Check sheet for the modelled part. Datum: model origin and axes. Units: mm. Face numbers are marked on the shaded views. A direction names the side the tool comes from. Round coordinates to 2 decimals unless told otherwise and drop trailing zeros. Write each loop counter-clockwise with the first axis right and the second up, starting at its lowest first coordinate (ties: lowest second). Pieces come first, ordered by that corner, then holes. Notation, with made-up numbers: (-20, -35.5) -> (34, -35.5) arc R19 ccw to (34, -11.5) -> close; hole circle Ø7 at (-21.75, 86). An arc over 180 degrees is marked (long way). One line per item, written item: value.
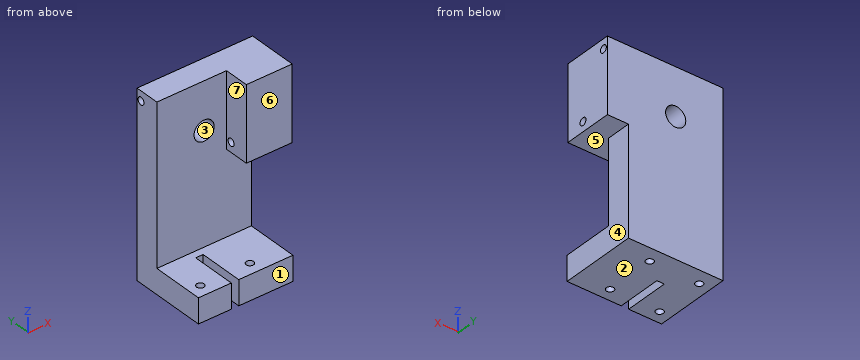
from build123d import *

# Parameters (mm, degrees)
SKETCH1_W                = 38.1
SKETCH1_H                = 63.5
SKETCH1_R                = 4.064
BOSS_EXTRUDE1_DEPTH      = 10
BOSS_EXTRUDE2_DEPTH      = 8.5
BOSS_EXTRUDE2_DEPTH_BACK = 10
BOSS_EXTRUDE2_START      = 38.1
SKETCH2_R                = 1.5
SKETCH3_R                = 1.5
BOSS_EXTRUDE3_DEPTH      = 10
SKETCH2_2_R              = 1.5
CUT_EXTRUDE1_DEPTH       = 10
CUT_EXTRUDE2_START       = 10
SKETCH3_2_R              = 1.5
CUT_EXTRUDE2_DEPTH       = 10


with BuildPart() as part:
    # Sketch1 → Boss-Extrude1 (new body)
    with BuildSketch(Plane(origin=(0, 0, 0), x_dir=(1, 0, 0), z_dir=(0, 1, 0))):
        with Locations((19.05, -31.75)):
            Rectangle(SKETCH1_W, SKETCH1_H)
        with Locations(Location((19.05, -44.45, 0), (0, 0, 270))):
            Circle(SKETCH1_R, mode=Mode.SUBTRACT)
    extrude(amount=BOSS_EXTRUDE1_DEPTH)

    # Sketch2 → Boss-Extrude2 (add, two sides: drawn at the far end of the back side and taken through both)
    with BuildSketch(Plane(origin=(0, 0, 0), x_dir=(0, 0, -1), z_dir=(1, 0, 0)).offset(BOSS_EXTRUDE2_START - BOSS_EXTRUDE2_DEPTH_BACK)):
        Polygon((-33.5, 0), (-33.5, -10), (-63.5, -10), (-63.5, 0), (-63.5, 10), (-33.5, 10), align=None)
        with Locations(Location((-59.6, 8, 0), (0, 0, 180))):
            Circle(SKETCH2_R, mode=Mode.SUBTRACT)
        with Locations(Location((-37.4, -2.3, 0), (0, 0, 180))):
            Circle(SKETCH2_R, mode=Mode.SUBTRACT)
    extrude(amount=BOSS_EXTRUDE2_DEPTH + BOSS_EXTRUDE2_DEPTH_BACK)

    # Sketch3 → Boss-Extrude3 (add)
    with BuildSketch(Plane.XY):
        Polygon((13.25, -21), (13.25, -3), (16.25, -3), (16.25, -21), (38.1, -21), (38.1, 10), (0, 10), (0, -21), align=None)
        with Locations((4.75, -16)):
            Circle(SKETCH3_R, mode=Mode.SUBTRACT)
        with Locations((24.75, -16)):
            Circle(SKETCH3_R, mode=Mode.SUBTRACT)
        with Locations((4.75, 4)):
            Circle(SKETCH3_R, mode=Mode.SUBTRACT)
        with Locations((24.75, 4)):
            Circle(SKETCH3_R, mode=Mode.SUBTRACT)
    extrude(amount=-BOSS_EXTRUDE3_DEPTH)

    # Sketch2<2> → Cut-Extrude1 (cut)
    with BuildSketch(Plane(origin=(0, 0, 0), x_dir=(0, 0, -1), z_dir=(1, 0, 0))):
        with Locations(Location((-59.6, 8, 0), (0, 0, 180))):
            Circle(SKETCH2_2_R)
    extrude(amount=CUT_EXTRUDE1_DEPTH, mode=Mode.SUBTRACT)

    # Sketch3<2> → Cut-Extrude2 (cut)
    with BuildSketch(Plane.XY.offset(CUT_EXTRUDE2_START)):
        with Locations((24.75, 4)):
            Circle(SKETCH3_2_R)
        with Locations((4.75, 4)):
            Circle(SKETCH3_2_R)
    extrude(amount=-CUT_EXTRUDE2_DEPTH, mode=Mode.SUBTRACT)


solid = part.part
Item 1: Tool access check on the marked faces 4, 5, 6 and 7. Record the directions out of +Z, -Z, +X, -X, +Y, -Y that give a thin tool (end or side, any length) a straight path to the whole face; none if there is none.
Answer:
face 4: -Z, +X, +Y, -Y
face 5: +X, -Y
face 6: +Z, +X, -X, -Y
face 7: +Z, -X, -Y
Item 2: Sectioned sample at B-B on y = -16. Enter the section's corners in (x, z).
Answer:
outline: (0, -10) -> (3.25, -10) -> (3.25, 0) -> (0, 0) -> close; (6.25, -10) -> (13.25, -10) -> (13.25, 0) -> (6.25, 0) -> close; (16.25, -10) -> (23.25, -10) -> (23.25, 0) -> (16.25, 0) -> close; (26.25, -10) -> (38.1, -10) -> (38.1, 0) -> (26.25, 0) -> close
Item 3: Thickness scan on line 1 (Y direction, x = 43, z = 59.6); line 2 (Y direction, x = 4.75, z = 0.5); line 3 (X direction, y = 6, z = 44.45). Record the ranges inside material, lowest first.
Answer:
line 1: y = -10 to 6.5, 9.5 to 10
line 2: y = 0 to 2.5, 5.5 to 10
line 3: x = 0 to 14.99, 23.11 to 46.6
Item 4: Depth check by flat-ended pin: P1, Ø12, axis at x = 35.5, y = -17, coming from the +Z side; P2, Ø3.5, axis at y = 8.5, z = 60, coming from the -X side; P3, Ø12, axis at x = 6.5, z = 34, coming from the -Y side; P4, Ø1.5, axis at x = 4.5, y = 3.5, coming from the -Z side. Enter the tip coordinate at first touch or a pass-through.
Answer:
P1: stops at z = 0
P2: stops at x = 0
P3: stops at y = 0
P4: stops at z = 10
Item 5: Sectioned sample at C-C on x = 31. Enter the section's corners in (y, z), and give its area (3 significant figures).
Answer:
outline: (-21, -10) -> (10, -10) -> (10, 63.5) -> (-10, 63.5) -> (-10, 33.5) -> (0, 33.5) -> (0, 0) -> (-21, 0) -> close; hole circle Ø3 at (-2.3, 37.4)
area: 1,240 mm^2
Item 6: Sectioned sample at D-D on y = -7. Enter the section's corners in (x, z), and give its area (3 significant figures).
Answer:
outline: (0, -10) -> (13.25, -10) -> (13.25, 0) -> (0, 0) -> close; (16.25, -10) -> (38.1, -10) -> (38.1, 0) -> (16.25, 0) -> close; (28.1, 33.5) -> (46.6, 33.5) -> (46.6, 63.5) -> (28.1, 63.5) -> close
area: 906 mm^2
Item 7: Sectioned sample at A-A on z = 37.4. Enter the section's corners in (x, y), and give its area (4 significant figures).
Answer:
outline: (0, 0) -> (28.1, 0) -> (28.1, -0.8) -> (46.6, -0.8) -> (46.6, 10) -> (0, 10) -> close; (28.1, -10) -> (46.6, -10) -> (46.6, -3.8) -> (28.1, -3.8) -> close
area: 595.5 mm^2
Item 8: Mould release check, pull along Z, two halves, no side actions. Record for the marked faces 1, 2 and 3: pulls with the +Z half, pulls with the -Z half, needs draft (parallel to the pull), parting line crosses it, or undercut.
Answer:
face 1: needs draft
face 2: pulls with the -Z half
face 3: undercut
